Geometry: see drawing. Coordinates: mm, zero at the bounding-box minimum. A direction names the side the tool comes from. Round coordinates to 2 decimals unless told otherwise and drop trailing zeros. Order: outer loops, then holes, each group sorted by start corner. A loop starts at its lowest first (then second) coordinate and runs counter-clockwise, first axis right, second up. Notation, with made-up numbers: (-20.75, 12.5) - (16.25, 12.5) arc R18 ccw to (16.25, 33.5) - close; hole circle Ø11 at (36.5, 77.25). An arc over 180 degrees is marked (long way). Put each result on its own line as item: value. Start each with the question number.
1) Mould query, pull axis X, two halves, no side actions, for the marked faces 1, 2 and 3. Classes: +X half, -X half, draft (parallel to the pull), parting line (faces both ways), or undercut.
2) Line query: probe 1 along X at (y, z) = (1.5, 17); probe 2 along Z at (x, y) = (1.75, 2.05); probe 3 along X at (y, z) = (1.2, 8.25). Output: solid intervals per line, ascending. Write a range as [from, to].
3) Section C-C on x = 12. Output: boundary loops of the cut face in (y, z), then the cut area to 3 significant figures.
4) Section D-D on z = 6. Output: boundary loops of the cut face in (x, y), then the cut area to 3 significant figures.
5) Section B-B on y = 1.33. Output: boundary loops of the cut face in (x, z).
6) Access query for the marked faces 4 and 5. Directions: +Z, -Z, +X, -X, +Y, -Y. A direction counts if a zero-diameter tool reaches every point of the face in a straight line with its end or side. Return the directions, or none.
7) Contact query for flat-ended pins moving along their axis: P1, Ø2.5, axis at x = 6, y = 1.5, coming from the +Z side; P2, Ø3, axis at x = 10.5, z = 4, coming from the -Y side; P3, Ø3, axis at y = 3, z = 8, coming from the -X side. Output: stop coordinate, or through.
8) Section A-A on z = 16.25. Output: boundary loops of the cut face in (x, y).
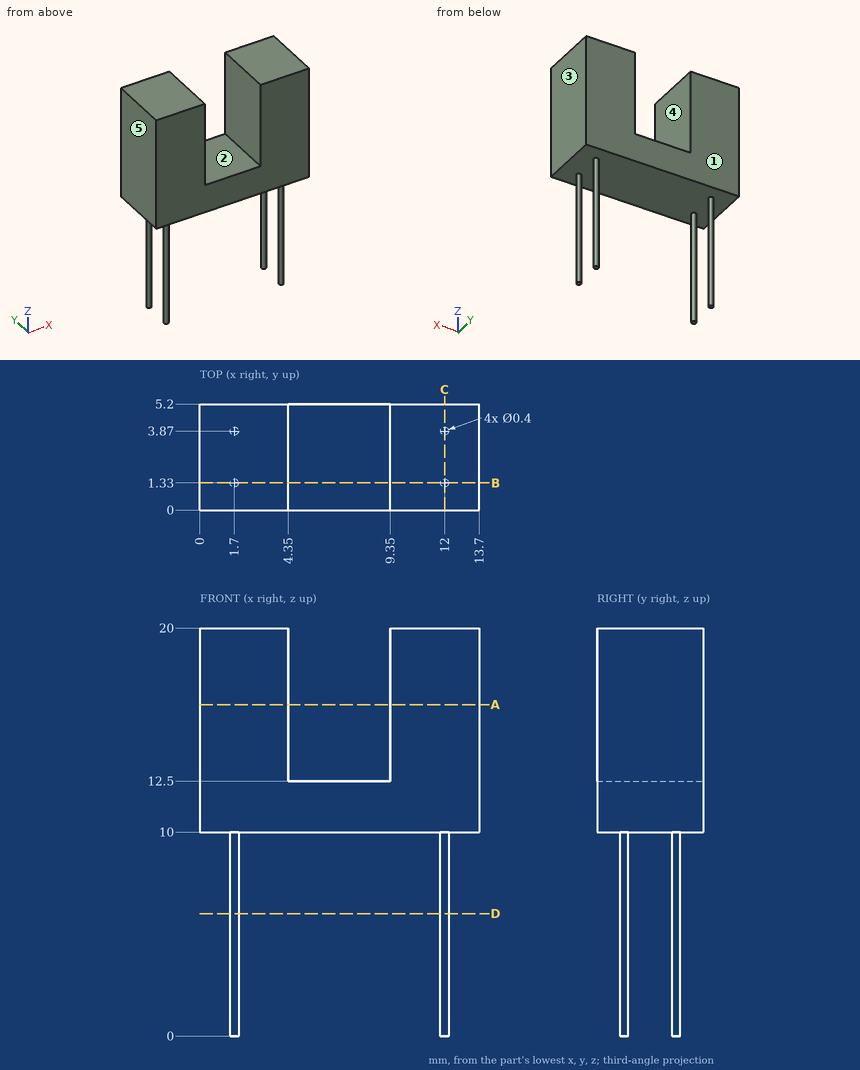
Answer sheet:
1. face 1: draft
1. face 2: undercut
1. face 3: +X half
2. probe 1: [0, 4.35], [9.35, 13.7]
2. probe 2: [10, 20]
2. probe 3: [1.55, 1.85], [11.85, 12.15]
3. outline: (0, 10) - (1.13, 10) - (1.13, 0) - (1.53, 0) - (1.53, 10) - (3.67, 10) - (3.67, 0) - (4.07, 0) - (4.07, 10) - (5.2, 10) - (5.2, 20) - (0, 20) - close
3. area: 60.0 mm^2
4. outline: circle Ø0.4 at (1.7, 1.33); circle Ø0.4 at (1.7, 3.87); circle Ø0.4 at (12, 1.33); circle Ø0.4 at (12, 3.87)
4. area: 0.503 mm^2
5. outline: (0, 10) - (1.5, 10) - (1.5, 0) - (1.9, 0) - (1.9, 10) - (11.8, 10) - (11.8, 0) - (12.2, 0) - (12.2, 10) - (13.7, 10) - (13.7, 20) - (9.35, 20) - (9.35, 12.5) - (4.35, 12.5) - (4.35, 20) - (0, 20) - close
6. face 4: +Z, +Y, -Y
6. face 5: +Z, -Z, -X, +Y, -Y
7. P1: z = 12.5
7. P2: y = 1.13
7. P3: x = 1.5
8. outline: (0, 0) - (4.35, 0) - (4.35, 5.2) - (0, 5.2) - close; (9.35, 0) - (13.7, 0) - (13.7, 5.2) - (9.35, 5.2) - close
